```python
from build123d import *

# Parameters (mm, degrees)
BOSS_EXTRUDE1_DEPTH = 5


with BuildPart() as part:
    # Sketch2 → Boss-Extrude1 (new body)
    with BuildSketch(Plane.XY.offset(324.609115736)):
        with BuildLine():
            Line((-16.90012844, -8.183190187), (72.816503584, -45.112441184))
            Line((72.816503584, -45.112441184), (83.47431689, -19.220144733))
            Line((83.47431689, -19.220144733), (-6.242315134, 17.709106264))
            add(Edge.make_bspline(
                [(-6.242315134, 17.709106264), (-19.147085678, 28.427579084), (-62.609683594, 83.624540664), (-113.341454038, 133.123455083), (-159.667254415, 160.823469136)],
                knots=[0, 0, 0, 0, 0.237148473, 1, 1, 1, 1], degree=3))
            add(Edge.make_bspline(
                [(-192.022205471, 204.724702407), (-183.525718419, 177.076811357), (-159.667254415, 160.823469136)],
                knots=[0, 0, 0, 1, 1, 1], degree=2))
            Line((-192.022205471, 204.724702407), (-204.287606756, 174.926900827))
            Line((-204.287606756, 174.926900827), (-208.911231122, 176.830081774))
            Line((-208.911231122, 176.830081774), (-219.569044429, 150.937785322))
            Line((-219.569044429, 150.937785322), (-214.945420062, 149.034604375))
            Line((-214.945420062, 149.034604375), (-224.18290752, 126.592874832))
            add(Edge.make_bspline(
                [(-175.911850273, 128.697068335), (-200.797987469, 136.066038881), (-224.18290752, 126.592874832)],
                knots=[0, 0, 0, 1, 1, 1], degree=2))
            add(Edge.make_bspline(
                [(-16.90012844, -8.183190187), (-30.222192507, 2.01197393), (-75.852029724, 55.431258283), (-128.517955825, 102.867060046), (-175.911850273, 128.697068335)],
                knots=[0, 0, 0, 0, 0.237148473, 1, 1, 1, 1], degree=3))
        make_face()
        with BuildLine():
            Line((65.049758472, -17.908345143), (-8.450005033, 12.345702))
            add(Edge.make_bspline(
                [(-8.450005033, 12.345702), (-21.566591824, 22.803900379), (-66.124581019, 77.120450197), (-117.836312175, 125.594689972), (-164.70691842, 152.362521961)],
                knots=[0, 0, 0, 0, 0.237148473, 1, 1, 1, 1], degree=3))
            ThreePointArc((-164.70691842, 152.362521961), (-175.410879134, 147.900994755), (-170.949351927, 137.19703404))
            add(Edge.make_bspline(
                [(-14.692438541, -2.819785922), (-27.809025332, 7.638412457), (-72.367014526, 61.954962275), (-124.078745683, 110.429202051), (-170.949351927, 137.19703404)],
                knots=[0, 0, 0, 0, 0.237148473, 1, 1, 1, 1], degree=3))
            Line((-14.692438541, -2.819785922), (58.807324964, -33.073833065))
            Line((58.807324964, -33.073833065), (65.049758472, -17.908345143))
        make_face(mode=Mode.SUBTRACT)
    extrude(amount=-BOSS_EXTRUDE1_DEPTH)


solid = part.part
```
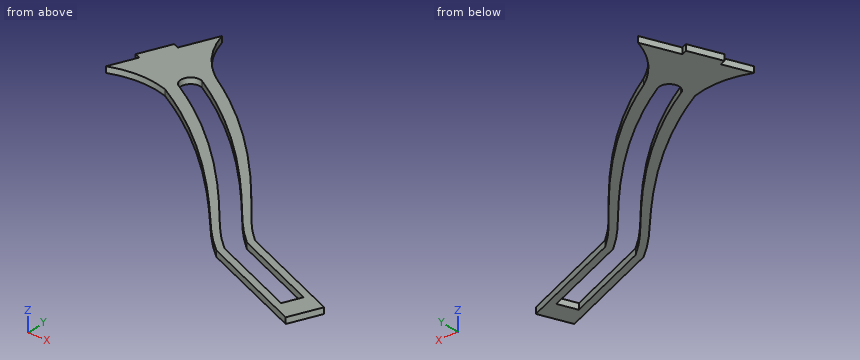
The model under review builds one solid part; all positions refer to its coordinate system, in mm. Round coordinates to 2 decimals unless told otherwise and drop trailing zeros. Loops run counter-clockwise (first coordinate to the right, second up) from the corner with the lowest first, then second, coordinate; pieces in that order, holes last. Notation, with made-up numbers: (57, 48.25) -> (73, 48.25) arc R22 ccw to (73, 84.25) -> close; hole circle Ø8 at (-19, 8.5). An arc over 180 degrees is marked (long way). Answer in a Markdown table with one row per item.
1) Consider section B-B, the plane x = 24. Write out the cut boundary in (y, z).
Taken from the geometry:
| item | result |
|---|---|
| outline | (-25.02, 319.61) -> (-18.75, 319.61) -> (-18.75, 324.61) -> (-25.02, 324.61) -> close; (-1.01, 319.61) -> (5.26, 319.61) -> (5.26, 324.61) -> (-1.01, 324.61) -> close |
2) For pin 1 Ø1 at (x, z) = (-94.5, 321) entering from +Y; pin 2 Ø3 at (y, z) = (178, 324) entering from -X, all flat-tipped, find the tip position at first contact; note any pin that passes through.
Taken from the geometry:
| item | result |
|---|---|
| pin 1 | stops at y = 112.14 |
| pin 2 | stops at x = -209.05 |
3) Wall thickness on line 1 along X through (y, z) = (3.5, 323.25); line 2 along X through (y, z) = (-12.5, 321.7); line 3 along Y through (x, z) = (-87, 322.35): over which ranges is each line inside the solid? List them lowest first.
Taken from the geometry:
| item | result |
|---|---|
| line 1 | x = -30.29 to -22.04, 13.04 to 28.28 |
| line 2 | x = -6.41 to 8.82, 51.91 to 67.15 |
| line 3 | y = 62.61 to 72.9, 94.01 to 104.66 |
4) Consider section A-A, the plane y = -11.5. Write out the cut boundary in (x, z), plus the area to 3 significant figures.
Taken from the geometry:
| item | result |
|---|---|
| outline | (-8.84, 319.61) -> (6.4, 319.61) -> (6.4, 324.61) -> (-8.84, 324.61) -> close; (49.48, 319.61) -> (64.72, 319.61) -> (64.72, 324.61) -> (49.48, 324.61) -> close |
| area | 152 mm² |
